Work out the finished part from the listing and answer in its coordinate system (mm). Face numbers are marked on the shaded views. A direction names the side the tool comes from. Give positions to 0.01 mm unless a question says otherwise; leave off trailing zeros. Loops run counter-clockwise (first coordinate to the right, second up) from the corner with the lowest first, then second, coordinate; pieces in that order, holes last.
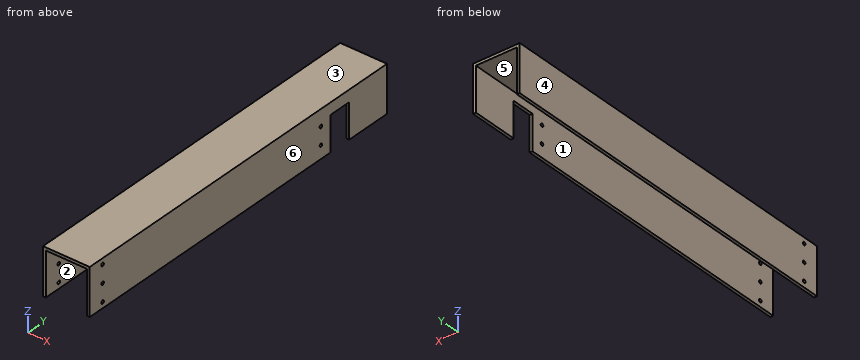
from build123d import *

# Parameters (mm, degrees)
BOSS_EXTRUDE1_DEPTH           = 400
SKETCH2_W                     = 3.175
SKETCH2_H                     = 25.4
CUT_EXTRUDE1_DEPTH            = 38.1
TAP_DRILL_FOR_8_32_TAP1_D     = 3.4544
TAP_DRILL_FOR_8_32_TAP2_D     = 3.4544
TAP_DRILL_FOR_8_32_TAP2_DEPTH = 3.175


with BuildPart() as part:
    # Sketch1 → Boss-Extrude1 (new body)
    with BuildSketch(Plane(origin=(0, 0, 0), x_dir=(1, 0, 0), z_dir=(0, 1, 0))):
        Polygon((0, 0), (0, -50.8), (50.8, -50.8), (50.8, 0), (47.625, 0), (47.625, -47.625), (3.175, -47.625), (3.175, 0), align=None)
    extrude(amount=BOSS_EXTRUDE1_DEPTH)

    # Sketch2 → Cut-Extrude1 (cut)
    with BuildSketch(Plane(origin=(0, 0, 0), x_dir=(-1, 0, 0), z_dir=(0, 0, -1))):
        with Locations((-49.2125, 336.5)):
            Rectangle(SKETCH2_W, SKETCH2_H)
    extrude(amount=-CUT_EXTRUDE1_DEPTH, mode=Mode.SUBTRACT)

    # Tap Drill for #8-32 Tap1 (through all)
    with Locations(Plane(origin=(50.8, 0, 0), x_dir=(0, 0, -1), z_dir=(1, 0, 0))):
        with Locations((-44.45, 17.3), (-25.4, 17.3), (-6.35, 17.3)):
            Hole(TAP_DRILL_FOR_8_32_TAP1_D / 2)

    # Tap Drill for #8-32 Tap2
    with Locations(Plane(origin=(50.8, 0, 0), x_dir=(0, 0, -1), z_dir=(1, 0, 0))):
        with Locations((-33.02, 311.1), (-13.97, 311.1)):
            Hole(TAP_DRILL_FOR_8_32_TAP2_D / 2, depth=TAP_DRILL_FOR_8_32_TAP2_DEPTH)


solid = part.part
Item 1: For the marked faces 5 and 6, determine the directions among +Z, -Z, +X, -X, +Y, -Y from which every point of the face is accessible in a straight line to the end or side of a thin tool.
Item 2: Flat-ended cylindrical pins translate along their axes: pin 1 Ø2 at (y, z) = (305.5, 7) entering from -X; pin 2 Ø3 at (y, z) = (17.3, 6.35) entering from -X; pin 3 Ø1 at (x, y) = (48.5, 340) entering from -Z; pin 4 Ø12 at (x, y) = (28.5, 50.5) entering from -Z (3 decimals). Find the tip coordinate at first contact, or state that the pin passes through.
Item 3: Find section A-A, the plane y = 227. Write down the section's boundary in (x, z) (3 decimals).
Item 4: Find section B-B, the plane x = 29. Write down the section's boundary in (y, z) (3 decimals).
Item 5: Consider line 1 (Z direction, x = 49, y = 311); line 2 (Y direction, x = 49, z = 13.97); line 3 (Z direction, x = 1, y = 17). Determine where each line is inside the solid, lowest interval first.
Item 6: Determine the mould class of the marked faces 1, 2, 3 and 4 for opening direction X: released by +X, released by -X, zero draft, split by the parting line, or undercut.
Ans:
1. face 5: -Z, +Y, -Y
1. face 6: +Z, -Z, +X, +Y, -Y
2. pin 1: stops at x = 0
2. pin 2: passes through
2. pin 3: stops at z = 38.1
2. pin 4: stops at z = 47.625
3. outline: (0, 0) - (3.175, 0) - (3.175, 47.625) - (47.625, 47.625) - (47.625, 0) - (50.8, 0) - (50.8, 50.8) - (0, 50.8) - close
4. outline: (0, 47.625) - (400, 47.625) - (400, 50.8) - (0, 50.8) - close
5. line 1: z = 0 to 12.25, 15.69 to 31.3, 34.74 to 50.8
5. line 2: y = 0 to 309.37, 312.83 to 323.8, 349.2 to 400
5. line 3: z = 0 to 4.65, 8.05 to 23.7, 27.1 to 42.75, 46.15 to 50.8
6. face 1: undercut
6. face 2: undercut
6. face 3: zero draft
6. face 4: released by -X
